```python
from build123d import *

# Parameters (mm, degrees)
SKETCH1_W                      = 142
SKETCH1_H                      = 82
BOSS_EXTRUDE1_DEPTH            = 5
M3_CLEARANCE_HOLE1_D           = 3.2
M3_CLEARANCE_HOLE1_CSINK_D     = 3.25
M3_CLEARANCE_HOLE1_CSINK_ANGLE = 90
FILLET1_R                      = 5


with BuildPart() as part:
    # Sketch1 → Boss-Extrude1 (new body)
    with BuildSketch(Plane(origin=(0, 0, 0), x_dir=(1, 0, 0), z_dir=(0, 1, 0))):
        Rectangle(SKETCH1_W, SKETCH1_H)
    extrude(amount=BOSS_EXTRUDE1_DEPTH)

    # M3 Clearance Hole1 (through all)
    with Locations(Plane(origin=(0, 5, 0), x_dir=(1, 0, 0), z_dir=(0, 1, 0))):
        with Locations((-63, 38), (-63, -38), (63, 38), (63, -38)):
            CounterSinkHole(M3_CLEARANCE_HOLE1_D / 2, M3_CLEARANCE_HOLE1_CSINK_D / 2, counter_sink_angle=M3_CLEARANCE_HOLE1_CSINK_ANGLE)

    # Fillet1
    fillet1_edges = [part.edges().sort_by_distance(p)[0] for p in [
        (71, 2.5, 41),
        (-71, 2.5, 41),
        (-71, 2.5, -41),
        (71, 2.5, -41),
    ]]
    fillet(fillet1_edges, radius=FILLET1_R)


solid = part.part
```
The model under review builds one solid part; all positions refer to its coordinate system, in mm. Round coordinates to 2 decimals unless told otherwise and drop trailing zeros. Loops run counter-clockwise (first coordinate to the right, second up) from the corner with the lowest first, then second, coordinate; pieces in that order, holes last. Notation, with made-up numbers: M 11,69.25 L 43,69.25 A17 ccw 43,83.25 Z; hole C 9.25,-37.75 d1. An arc over 180 degrees is marked long. Put each result on its own line as item: value.
Q1. Mouldability with a two-part tool opening along Z and no side actions: class faces 1 (the cylindrical face through (-63.74, 2.45, 39.42)), 2 (the cylindrical face through (-70, 3, -39)), 3 (the cylindrical face through (70, 3, 39)), 4 (the flat face through (-71, 2, 1)) as released by +Z, released by -Z, zero draft, split by the parting line, or undercut.
Result set:
face 1: undercut
face 2: released by -Z
face 3: released by +Z
face 4: zero draft
Q2. Consider section B-B, the plane z = 38. Give the boundary of the cut face in (x, y) (3 decimals).
Result set:
outline: M -70.583,0 L -64.6,0 L -64.6,4.975 L -64.625,5 L -70.583,5 Z; M -61.4,0 L 61.4,0 L 61.4,4.975 L 61.375,5 L -61.375,5 L -61.4,4.975 Z; M 64.6,0 L 70.583,0 L 70.583,5 L 64.625,5 L 64.6,4.975 Z
Q3. To check wall thickness, follow L1, parallel to Z at x = 63, y = 1.4; L2, parallel to X at y = 1.2, z = 38; L3, parallel to Z at x = -64, y = 3.15. State the ranges of each line that lie inside material, in increasing order.
Result set:
L1: z = -41 to -39.6, -36.4 to 36.4, 39.6 to 41
L2: x = -70.58 to -64.6, -61.4 to 61.4, 64.6 to 70.58
L3: z = -41 to -39.25, -36.75 to 36.75, 39.25 to 41
Q4. For pin 1 (3 mm diameter, centred on x = 63, z = 38, fed in from +Y), flat-tipped, find the tip position at first contact; note if it passes through.
Result set:
pin 1: passes through
Q5. Consider section A-A, the plane x = -63. Give the boundary of the cut face in (y, z) (3 decimals), then the cut area to 3 significant figures.
Result set:
outline: M 0,-41 L 5,-41 L 5,-39.625 L 4.975,-39.6 L 0,-39.6 Z; M 0,-36.4 L 4.975,-36.4 L 5,-36.375 L 5,36.375 L 4.975,36.4 L 0,36.4 Z; M 0,39.6 L 4.975,39.6 L 5,39.625 L 5,41 L 0,41 Z
area: 378 mm²
